from build123d import *

# Parameters (mm, degrees)
F1_DEPTH = 9.525
F3_R     = 6.35
F4_DEPTH = 50.8
F5_SIZE  = 5.08
F6_SIZE  = 1.27


with BuildPart() as f1:
    # F0 (on Front) → F1 (new body)
    with BuildSketch(Plane.XZ):
        Polygon((-1.610126, 10.880027), (-10.227443, 4.045603), (-8.617317, -6.834424), (1.610126, -10.880027), (10.227443, -4.045603), (8.617317, 6.834424), align=None)
    extrude(amount=F1_DEPTH)

    # F3 (on offset) → F4 (join)
    with BuildSketch(Plane(origin=(0, 0, 0), x_dir=(1, 0, 0), z_dir=(0, 1, 0))):
        Circle(F3_R)
    extrude(amount=F4_DEPTH)

    # F5
    f5_edges = [f1.edges().sort_by_distance(p)[0] for p in [
        (-6.35, 50.8, 0),
    ]]
    chamfer(f5_edges, length=F5_SIZE)

    # F6
    f6_edges = [f1.edges().sort_by_distance(p)[0] for p in [
        (-5.918785, -9.525, 7.462815),
        (3.503595, -9.525, 8.857226),
        (9.42238, -9.525, 1.39441),
        (5.918785, -9.525, -7.462815),
        (-3.503595, -9.525, -8.857226),
        (-9.42238, -9.525, -1.39441),
    ]]
    chamfer(f6_edges, length=F6_SIZE)


solid = f1.part
Geometry check sheet. Reference: the model listing, model coordinates, mm. A direction names the side the tool comes from. Coordinates: 2 decimals unless noted, no trailing zeros. Write each loop counter-clockwise with the first axis right and the second up, starting at its lowest first coordinate (ties: lowest second). Pieces come first, ordered by that corner, then holes. Notation, with made-up numbers: (-26, 58) -> (28, 58) arc R23 cw to (28, 94) -> close; hole circle Ø4 at (86, 32.5). An arc over 180 degrees is marked (long way). One line per question, with ' | ' between items.
1. Cross-section at B-B on y = 39. Record the cut outline in (x, z).
Answers:
outline: circle Ø12.7 at (0, 0)
2. Cross-section at A-A on z = 0. Record the cut outline in (x, y) (3 decimals), and give its area (3 significant figures).
Answers:
outline: (-9.629, -8.255) -> (-8.345, -9.525) -> (8.345, -9.525) -> (9.629, -8.255) -> (9.629, 0) -> (6.35, 0) -> (6.35, 45.72) -> (1.27, 50.8) -> (-1.27, 50.8) -> (-6.35, 45.72) -> (-6.35, 0) -> (-9.629, 0) -> close | area: 801 mm²
3. Set-up check for faces 1 (the flat face through (-5.458, -8.899, 7.006)), 2 (the cylindrical face through (-1.38, 22.54, 6.2)): record each of +Z, -Z, +X, -X, +Y, -Y from which the full face is reachable in a straight line by a thin tool's end or side.
Answers:
face 1: +Z, -X, -Y | face 2: +Y
4. Depth check by flat-ended pin: pin 1 Ø1 at (x, z) = (-8, -7) entering from +Y; pin 2 Ø6 at (x, y) = (7, 3.5) entering from -Z; pin 3 Ø1.5 at (x, y) = (3, 22) entering from -Z. Enter the tip coordinate at first touch or a pass-through.
Answers:
pin 1: stops at y = 0 | pin 2: stops at z = -4.93 | pin 3: stops at z = -5.94
5. Cross-section at C-C on x = 0. Record the cut outline in (y, z) (3 decimals), and give its area (3 significant figures).
Answers:
outline: (-9.525, -8.877) -> (-8.255, -10.243) -> (0, -10.243) -> (0, -6.35) -> (45.72, -6.35) -> (50.8, -1.27) -> (50.8, 1.27) -> (45.72, 6.35) -> (0, 6.35) -> (0, 10.243) -> (-8.255, 10.243) -> (-9.525, 8.877) -> close | area: 813 mm²
6. Thickness scan on probe 1 along Y at (x, z) = (5, -4.25) (3 decimals); probe 2 along Z at (x, y) = (0, 11); probe 3 along Z at (x, y) = (-2.25, 10). Record the ranges inside material, lowest first. Write a range as from..to.
Answers:
probe 1: y = -9.525..0 | probe 2: z = -6.35..6.35 | probe 3: z = -5.94..5.94
